from build123d import *

# Parameters (mm, degrees)
F0_R     = 3.81
F1_DEPTH = 38.1
F3_DEPTH = 19.05


with BuildPart() as f1:
    # F0 (on Front) → F1 (new body)
    with BuildSketch(Plane.XZ):
        with BuildLine():
            Line((-31.75, -6.35), (38.1, -6.35))
            Line((38.1, -6.35), (38.1, 0))
            Line((38.1, 0), (-25.4, 0))
            ThreePointArc((-25.4, 0), (-27.259872, -4.490128), (-31.75, -6.35))
        make_face()
        with Locations((-31.75, 0)):
            Circle(F0_R)
        with BuildLine():
            ThreePointArc((-25.4, 0), (-36.240128, 4.490128), (-31.75, -6.35))
            ThreePointArc((-31.75, -6.35), (-27.259872, -4.490128), (-25.4, 0))
        make_face()
        with Locations((-31.75, 0)):
            Circle(F0_R, mode=Mode.SUBTRACT)
    extrude(amount=F1_DEPTH)

    # F2 (on face) → F3 (cut)
    with BuildSketch(Plane.XZ.offset(38.1)):
        with BuildLine():
            Line((-25.4, -6.35), (-25.4, 0))
            ThreePointArc((-25.4, 0), (-36.240128, 4.490128), (-31.75, -6.35))
            Line((-31.75, -6.35), (-25.4, -6.35))
        make_face()
    extrude(amount=-F3_DEPTH, mode=Mode.SUBTRACT)


solid = f1.part
The listing builds one solid part. Answer for the finished solid, in the listing's coordinates (mm). A direction names the side the tool comes from. Round coordinates to 2 decimals unless told otherwise and drop trailing zeros. Write each loop counter-clockwise with the first axis right and the second up, starting at its lowest first coordinate (ties: lowest second). Pieces come first, ordered by that corner, then holes. Notation, with made-up numbers: (20, 38.5) - (54, 38.5) arc R31 cw to (54, 68.5) - close; hole circle Ø7 at (26, -3). An arc over 180 degrees is marked (long way). Use a Markdown table: item, result. Add a question column.
1. The part is cut by section C-C (x = -16.5). Write down the section's boundary in (y, z), and give its area (3 significant figures).
2. The part is cut by section B-B (y = -3). Write down the section's boundary in (x, z), and give its area (3 significant figures).
3. For a pull along Z with two mould halves and no side action, classify faces 3 (the face through (3, -19, -6.35)), 4 (the face through (7, -19, 0)), 5 (the face through (-1, 0, -3)), 6 (the face through (-28.23, -9.39, -1.46)) as +Z half, -Z half, draft (parallel to the pull), parting line (faces both ways), or undercut.
4. Flat-ended cylindrical pins translate along their axes: P1, Ø3, axis at y = -33.5, z = -3.5, coming from the -X side; P2, Ø1.5, axis at y = -25.5, z = 2, coming from the +X side; P3, Ø5, axis at y = -17, z = 4, coming from the -X side; P4, Ø4, axis at x = 20, y = -19, coming from the +Z side. Find the tip coordinate at first contact, or state that the pin passes through.
5. Consider line 1 (Z direction, x = -31.75, y = -13.25); line 2 (X direction, y = -8.5, z = -1.75); line 3 (Z direction, x = 30.5, y = -25). Determine where each line is inside the solid, lowest interval first.
6. The part is cut by section D-D (y = -34). Write down the section's boundary in (x, z), and give its area (3 significant figures).
7. The part is cut by section A-A (z = -2). Write down the section's boundary in (x, y), and give its area (3 significant figures).
8. A tool of negligible diameter and unlimited length cuts with its end or side. For faces 1 (the face through (-29, -19.05, -3)), 2 (the face through (38.1, -19, -3)), from which of +Z, -Z, +X, -X, +Y, -Y can it reach the whole face along a straight path? Write none if from no direction.
Reported:
| question | item | result |
|---|---|---|
| 1 | outline | (-38.1, -6.35) - (0, -6.35) - (0, 0) - (-38.1, 0) - close |
| 1 | area | 242 mm^2 |
| 2 | outline | (-31.75, -6.35) - (38.1, -6.35) - (38.1, 0) - (-25.4, 0) arc R6.35 ccw (long way) to start; hole circle Ø7.62 at (-31.75, 0) |
| 2 | area | 493 mm^2 |
| 3 | face 3 | -Z half |
| 3 | face 4 | +Z half |
| 3 | face 5 | draft |
| 3 | face 6 | undercut |
| 4 | P1 | x = -25.4 |
| 4 | P2 | through |
| 4 | P3 | x = -37.92 |
| 4 | P4 | z = 0 |
| 5 | line 1 | -6.35 to -3.81, 3.81 to 6.35 |
| 5 | line 2 | -37.85 to -35.13, -28.37 to 38.1 |
| 5 | line 3 | -6.35 to 0 |
| 6 | outline | (-25.4, -6.35) - (38.1, -6.35) - (38.1, 0) - (-25.4, 0) - close |
| 6 | area | 403 mm^2 |
| 7 | outline | (-37.78, -19.05) - (-34.99, -19.05) - (-34.99, 0) - (-37.78, 0) - close; (-28.51, -19.05) - (-25.4, -19.05) - (-25.4, -38.1) - (38.1, -38.1) - (38.1, 0) - (-28.51, 0) - close |
| 7 | area | 2,530 mm^2 |
| 8 | face 1 | +Z, -Z, -X, -Y |
| 8 | face 2 | +Z, -Z, +X, +Y, -Y |
